from build123d import *

# Parameters (mm, degrees)
SKETCH2_R     = 0.762
CHAMFER1_SIZE = 0.381
FILLET1_R     = 0.508
CHAMFER2_SIZE = 0.381


with BuildPart() as part:
    # Sketch1 → Revolve1 (revolve)
    with BuildSketch(Plane.XY, mode=Mode.PRIVATE) as revolve1_sk:
        Polygon((2.413, -6.35), (6.35, -6.35), (6.35, 0), (14.2875, 0), (14.2875, 12.7), (11.1125, 12.7), (2.413, 4.0005), align=None)
    revolve(revolve1_sk.sketch.rotate(Axis((0, 0, 0), (0, 1, 0)), 90), axis=Axis((0, 0, 0), (0, 1, 0)))  # turned: the seam where the file's is

    # Sketch2 → Cut-Revolve1 (revolve, cut)
    with BuildSketch(Plane.XY, mode=Mode.PRIVATE) as cut_revolve1_sk:
        with Locations((6.858, -0.508)):
            Circle(SKETCH2_R)
    revolve(cut_revolve1_sk.sketch.rotate(Axis((0, 0, 0), (0, -1, 0)), 270), axis=Axis((0, 0, 0), (0, -1, 0)), mode=Mode.SUBTRACT)  # turned: the seam where the file's is

    # Chamfer1
    chamfer1_edges = [part.edges().sort_by_distance(p)[0] for p in [
        (0, -6.35, 2.413),
    ]]
    chamfer(chamfer1_edges, length=CHAMFER1_SIZE)

    # Fillet1
    fillet1_edges = [part.edges().sort_by_distance(p)[0] for p in [
        (0, 0, 14.2875),
        (0, 12.7, 14.2875),
        (0, 12.7, 11.1125),
    ]]
    fillet(fillet1_edges, radius=FILLET1_R)

    # Chamfer2
    chamfer2_edges = [part.edges().sort_by_distance(p)[0] for p in [
        (0, -6.35, 6.35),
    ]]
    chamfer(chamfer2_edges, length=CHAMFER2_SIZE)


solid = part.part
Source: CAD feature listing. Evaluate the final solid. Frame: model axes, mm. A direction names the side the tool comes from. Round coordinates to 2 decimals unless told otherwise and drop trailing zeros. Loops run counter-clockwise (first coordinate to the right, second up) from the corner with the lowest first, then second, coordinate; pieces in that order, holes last. Notation, with made-up numbers: (48, -39) -> (82, -39) arc R3 cw to (82, -35) -> close; hole circle Ø2 at (60, 52.25). An arc over 180 degrees is marked (long way). Answer as a JSON object with one key per item and string values. Group by question number.
Q1. Section query B-B (z = 0). Output: boundary loops of the cut face in (x, y).
Q2. Section query A-A (x = 0). Output: boundary loops of the cut face in (y, z), plus the area to 3 significant figures.
Q3. Access query for faces 1 (the cylindrical face through (1.468, -1.054, 1.915)), 2 (the flat face through (6, 0, 6)). Directions: +Z, -Z, +X, -X, +Y, -Y. A direction counts if a zero-diameter tool reaches every point of the face in a straight line with its end or side. Return the directions, or none.
Q4. Mould query, pull axis X, two halves, no side actions, for faces 3 (the flat face through (3, -6.35, 1)), 4 (the cylindrical face through (-0.628, 6.432, 14.274)), 5 (the conical face through (-3.75, 5.37, 0.49)). Classes: pulls with the +X half, pulls with the -X half, needs draft (parallel to the pull), parting line crosses it, or undercut.
Q5. Ray query, line 1 (X direction, y = -1.5, z = 0); line 2 (X direction, y = 1.75, z = 0); line 3 (Y direction, x = 8.5, z = 7.5). Return the intervals inside material, ascending. Write a range as from..to.
Q6. Section query C-C (y = -2). Output: boundary loops of the cut face in (x, z).
Q7. Section query D-D (y = 7.5). Output: boundary loops of the cut face in (x, z) (1 decimal).
Q8. Contact query for flat-ended pins moving along their axis: P1, Ø2, axis at x = 11, y = 2, coming from the -Z side; P2, Ø1.5, axis at y = 1, z = -7.5, coming from the +X side; P3, Ø8, axis at x = -3.5, z = 1, coming from the +Y side. Output: stop coordinate, or through.
Completed:
{
 "1": {"outline": "(-14.29, 0.51) arc R0.51 ccw to (-13.78, 0) -> (-7.43, 0) arc R0.76 cw (long way) to (-6.35, -1.08) -> (-6.35, -5.97) -> (-5.97, -6.35) -> (-2.79, -6.35) -> (-2.41, -5.97) -> (-2.41, 4) -> (-10.96, 12.55) arc R0.51 ccw to (-11.32, 12.7) -> (-13.78, 12.7) arc R0.51 ccw to (-14.29, 12.19) -> close; (2.41, -5.97) -> (2.79, -6.35) -> (5.97, -6.35) -> (6.35, -5.97) -> (6.35, -1.08) arc R0.76 cw (long way) to (7.43, 0) -> (13.78, 0) arc R0.51 ccw to (14.29, 0.51) -> (14.29, 12.19) arc R0.51 ccw to (13.78, 12.7) -> (11.32, 12.7) arc R0.51 ccw to (10.96, 12.55) -> (2.41, 4) -> close"},
 "2": {"outline": "(-6.35, -5.97) -> (-5.97, -6.35) -> (-1.08, -6.35) arc R0.76 cw (long way) to (0, -7.43) -> (0, -13.78) arc R0.51 ccw to (0.51, -14.29) -> (12.19, -14.29) arc R0.51 ccw to (12.7, -13.78) -> (12.7, -11.32) arc R0.51 ccw to (12.55, -10.96) -> (4, -2.41) -> (-5.97, -2.41) -> (-6.35, -2.79) -> close; (-6.35, 2.79) -> (-5.97, 2.41) -> (4, 2.41) -> (12.55, 10.96) arc R0.51 ccw to (12.7, 11.32) -> (12.7, 13.78) arc R0.51 ccw to (12.19, 14.29) -> (0.51, 14.29) arc R0.51 ccw to (0, 13.78) -> (0, 7.43) arc R0.76 cw (long way) to (-1.08, 6.35) -> (-5.97, 6.35) -> (-6.35, 5.97) -> close", "area": "275 mm²"},
 "3": {"face 1": "+Y, -Y", "face 2": "-Y"},
 "4": {"face 3": "needs draft", "face 4": "parting line crosses it", "face 5": "undercut"},
 "5": {"line 1": "-6.35..-2.41, 2.41..6.35", "line 2": "-14.29..-2.41, 2.41..14.29", "line 3": "0..12.7"},
 "6": {"outline": "circle Ø12.7 at (0, 0); hole circle Ø4.83 at (0, 0)"},
 "7": {"outline": "circle Ø28.6 at (0, 0); hole circle Ø11.8 at (0, 0)"},
 "8": {"P1": "z = -10.2", "P2": "x = 12.59", "P3": "y = 9.23"}
}
